Autodesk Inventor part; units mm, degrees
ref_plane "YZ Plane" through (0, 0, 0) normal (1, 0, 0) x (0, 1, 0)
ref_plane "XZ Plane" through (0, 0, 0) normal (0, 1, 0) x (-1, 0, 0)
ref_plane "XY Plane" through (0, 0, 0) normal (0, 0, 1) x (1, 0, 0)
sketch "Sketch_1" plane through (0, 0, 0) normal (1, 0, 0) x (0, 1, 0)
  line L0 (2.3431, 60) -> (0, 60)
  line L1 (0, 60) -> (0, 0)
  line L2 (0, 0) -> (60, 0)
  line L3 (60, 0) -> (60, 2.3431)
  arc A0 (60, 2.3431) -> (58.8284, 5.1716) centre (56, 2.3431) ccw
  line L4 (58.8284, 5.1716) -> (5.1716, 58.8284)
  arc A1 (5.1716, 58.8284) -> (2.3431, 60) centre (2.3431, 56) ccw
  line L5 (4, 54.3431) -> (4, 4)
  line L6 (4, 4) -> (54.3431, 4)
  line L7 (54.3431, 4) -> (4, 54.3431)
extrude "Extrusion1" add sketch "Sketch_1" along normal mid plane 27
sketch "Sketch2" plane through (-13.5, 0, 0) normal (0, -1, 0) x (1, 0, 0)
  point P0 (13.5, 15)
hole "Hole1" at (0, 0, 15) direction (0, 1, 0) diameter 6.81 depth 4
sketch "Sketch3" plane through (13.5, 60, 0) normal (0, 0, -1) x (-1, 0, 0)
  point P0 (13.5, -45)
hole "Hole2" at (0, 15, 0) direction (0, 0, 1) diameter 6.81 depth 4
sketch "Sketch_4" plane through (0, 0, 60) normal (0, 0, 1) x (1, 0, 0)
  circle A0 centre (0, 15) radius 6.35
extrude "Extrusion2" cut sketch "Sketch_4" against normal blind 56
sketch "Sketch_5" plane through (0, 60, 0) normal (0, 1, 0) x (1, 0, 0)
  circle A0 centre (0, -15) radius 6.35
extrude "Extrusion3" cut sketch "Sketch_5" against normal blind 56
sketch "Sketch6" plane through (13.5, 60, 0) normal (0, 0, -1) x (-1, 0, 0)
  point P0 (13.5, -15)
hole "Hole3" at (0, 45, 0) direction (0, 0, 1) diameter 6.81 depth 4
sketch "Sketch7" plane through (-13.5, 0, 0) normal (0, -1, 0) x (1, 0, 0)
  point P0 (13.5, 45)
hole "Hole4" at (0, 0, 45) direction (0, 1, 0) diameter 6.81 depth 4
sketch "Sketch_8" plane through (0, 0, 60) normal (0, 0, 1) x (1, 0, 0)
  circle A0 centre (0, 45) radius 6.35
extrude "Extrusion4" cut sketch "Sketch_8" against normal blind 56
sketch "Sketch_9" plane through (0, 60, 0) normal (0, 1, 0) x (1, 0, 0)
  circle A0 centre (0, -45) radius 6.35
extrude "Extrusion5" cut sketch "Sketch_9" against normal blind 56
properties part number "30-4336 Aluminum"
Part model, mm, in its own coordinate system. A direction names the side the tool comes from. Give positions to 0.01 mm unless a question says otherwise; leave off trailing zeros. Loops run counter-clockwise (first coordinate to the right, second up) from the corner with the lowest first, then second, coordinate; pieces in that order, holes last. Notation, with made-up numbers: (45.5, 28) -> (82.5, 28) arc R23 cw to (82.5, 65) -> close; hole circle Ø3 at (21.5, 65). An arc over 180 degrees is marked (long way). Write each question's results on one line, items separated by ' | '. Start each with the question number.
Q1. Band-saw the part on D-D on x = 0. Count the separate pieces of the cut face and the enclosed holes in it, plus the area to 3 significant figures.
Q2. Band-saw the part on B-B on x = 8. List the corners of the cut face in (y, z).
Q3. Pin check, flat tips, straight feed: P1, Ø12, axis at x = -2.5, z = 50, coming from the +Y side; P2, Ø7.5, axis at x = 0, y = 15, coming from the +Z side; P3, Ø2, axis at x = 6.5, y = 16.5, coming from the +Z side. Stop position of each tip, or through.
Q4. Pull direction Z, two halves, no side cores. Call faces 1 (the face through (0.748, 8.338, 51.306)), 2 (the face through (0, 1, 60)), 3 (the face through (-13.5, 28, 32)): +Z half, -Z half, draft (parallel to the pull), parting line (faces both ways), or undercut.
Q5. Which spindle directions (+Z, -Z, +X, -X, +Y, -Y) get a long thin tool onto all of the face, cutting with end or side? Do faces 4 (the face through (0.748, 38.338, 21.306)), 5 (the face through (0, 29, 4)), 6 (the face through (-0.06, 8.65, 51.75)). Say none if no direction does.
Q6. Band-saw the part on C-C on z = 31. List the corners of the cut face in (x, y), plus the area to 3 significant figures.
Q7. Band-saw the part on A-A on z = 46. List the corners of the cut face in (x, y), plus the area to 3 significant figures.
Q8. Wall check: L1, parallel to X at y = 1, z = 45 (3 decimals); L2, parallel to Y at x = -3.75, z = 57; L3, parallel to Z at x = -2.5, y = 24. Give the ranges that are in metal, low to high.
Results are:
1) separate pieces: 6 | enclosed holes: 0 | area: 493 mm²
2) outline: (0, 0) -> (60, 0) -> (60, 2.34) arc R4 ccw to (58.83, 5.17) -> (5.17, 58.83) arc R4 ccw to (2.34, 60) -> (0, 60) -> close; hole (4, 4) -> (54.34, 4) -> (4, 54.34) -> close
3) P1: stops at y = 18.61 | P2: stops at z = 4 | P3: stops at z = 48.5
4) face 1: undercut | face 2: +Z half | face 3: draft
5) face 4: +Y | face 5: +X, -X | face 6: +Z
6) outline: (-13.5, 0) -> (13.5, 0) -> (13.5, 4) -> (-13.5, 4) -> close; (-13.5, 27.34) -> (13.5, 27.34) -> (13.5, 33) -> (-13.5, 33) -> close | area: 261 mm²
7) outline: (-13.5, 0) -> (-3.25, 0) -> (-3.25, 4) -> (-13.5, 4) -> close; (-13.5, 12.34) -> (-6.27, 12.34) -> (-6.27, 14) arc R6.35 cw to (-6.27, 16) -> (-6.27, 18) -> (-13.5, 18) -> close; (3.25, 0) -> (13.5, 0) -> (13.5, 4) -> (3.25, 4) -> close; (6.27, 12.34) -> (13.5, 12.34) -> (13.5, 18) -> (6.27, 18) -> (6.27, 16) arc R6.35 cw to (6.27, 14) -> close | area: 164 mm²
8) L1: x = -13.5 to -3.405, 3.405 to 13.5 | L2: y = 0 to 7 | L3: z = 0 to 4, 34.34 to 39.16
